```python
from build123d import *

# Parameters (mm, degrees)
BOSS_EXTRUDE1_DEPTH         = 12.7
SKETCH2_W                   = 323.85
SKETCH2_H                   = 152.4
CUT_EXTRUDE1_DEPTH          = 12.7
F_1_4_0_25_DIAMETER_HOLE1_D = 6.35
CUT_EXTRUDE2_DEPTH          = 13.7
SKETCH9_R                   = 3.175
CUT_EXTRUDE3_DEPTH          = 13.7
SKETCH10_R                  = 3.175
CUT_EXTRUDE4_DEPTH          = 13.7
LPATTERN1_COUNT             = 5
LPATTERN1_PITCH             = 25.4


with BuildPart() as part:
    # Sketch1 → Boss-Extrude1 (new body)
    with BuildSketch(Plane(origin=(0, 0, 0), x_dir=(0, 0, -1), z_dir=(1, 0, 0))):
        with BuildLine():
            Line((0, 609.6), (323.85, 609.6))
            Line((323.85, 609.6), (323.85, 0))
            Line((323.85, 0), (0, 0))
            Line((0, 0), (0, 31.75))
            ThreePointArc((0, 31.75), (188.340145046, 304.8), (0, 577.85))
            Line((0, 577.85), (0, 609.6))
        make_face()
    extrude(amount=BOSS_EXTRUDE1_DEPTH)

    # Sketch2 → Cut-Extrude1 (cut)
    with BuildSketch(Plane(origin=(12.7, 0, 0), x_dir=(0, 0, -1), z_dir=(1, 0, 0))):
        with Locations((161.925, 533.4)):
            Rectangle(SKETCH2_W, SKETCH2_H)
    extrude(amount=-CUT_EXTRUDE1_DEPTH, mode=Mode.SUBTRACT)

    # 1/4 (0.25) Diameter Hole1 (through all)
    with Locations(Plane(origin=(12.7, 0, 0), x_dir=(0, 0, -1), z_dir=(1, 0, 0))):
        with Locations((20.67422398, 12.7), (44.370645325, 23.973354386), (67.055185152, 37.165039515), (88.57288505, 52.184942803), (108.776757311, 68.93046308), (127.528789002, 87.287211463), (144.70088473, 107.129792746), (160.17574167, 128.32266198), (173.847650859, 150.721050378), (185.623219292, 174.171954236), (195.422007898, 198.515180102), (203.177081014, 223.584439059), (208.835463627, 249.208482649), (212.358503247, 275.212272671), (213.722133941, 301.418176873), (212.917040728, 327.647182356), (209.948723211, 353.720118416), (204.837458009, 379.458880463), (197.618160246, 404.687646654), (188.340145046, 429.234078933)):
            Hole(F_1_4_0_25_DIAMETER_HOLE1_D / 2)

    # Sketch8 → Cut-Extrude2 (cut, through all)
    with BuildSketch(Plane(origin=(12.7, 0, 0), x_dir=(0, 0, -1), z_dir=(1, 0, 0))):
        with BuildLine():
            Line((270.760801555, 457.2), (323.85, 457.2))
            Line((323.85, 457.2), (323.85, 0))
            Line((323.85, 0), (161.925, 0))
            ThreePointArc((161.925, 0), (289.589524386, 211.163746738), (270.760801555, 457.2))
        make_face()
    extrude(amount=-CUT_EXTRUDE2_DEPTH, mode=Mode.SUBTRACT)

    # Sketch9 → Cut-Extrude3 (cut, through all)
    with BuildSketch(Plane(origin=(12.7, 0, 0), x_dir=(0, 0, -1), z_dir=(1, 0, 0))):
        with Locations((214.065703753, 83.37972827)):
            Circle(SKETCH9_R)
        with Locations((277.383754924, 373.862081852)):
            Circle(SKETCH9_R)
    extrude(amount=-CUT_EXTRUDE3_DEPTH, mode=Mode.SUBTRACT)

    # Sketch10 → Cut-Extrude4 (cut, through all)
    with BuildSketch(Plane.ZY):
        with Locations((-154.03800305, 12.7)):
            Circle(SKETCH10_R)
    cut_extrude4 = extrude(amount=-CUT_EXTRUDE4_DEPTH, mode=Mode.SUBTRACT)

    # LPattern1: Cut-Extrude4 ×5
    with Locations(*[(0, 0, i * LPATTERN1_PITCH) for i in range(1, LPATTERN1_COUNT)]):
        add(cut_extrude4, mode=Mode.SUBTRACT)


solid = part.part
```
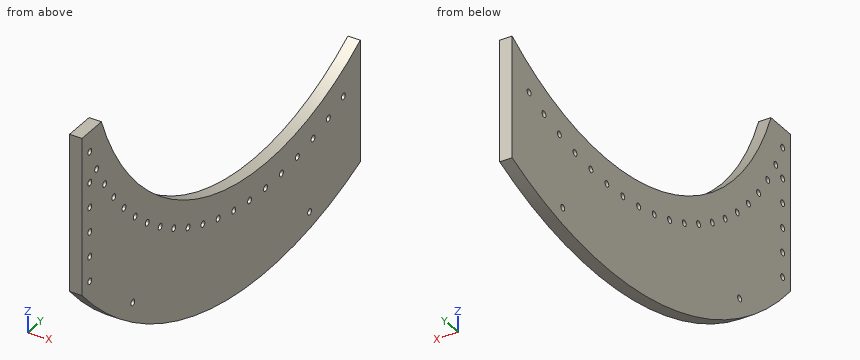
The model under review builds one solid part; all positions refer to its coordinate system, in mm. Round coordinates to 2 decimals unless told otherwise and drop trailing zeros. Write each loop counter-clockwise with the first axis right and the second up, starting at its lowest first coordinate (ties: lowest second). Pieces come first, ordered by that corner, then holes. Notation, with made-up numbers: (11, 5) - (33, 5) arc R23 cw to (33, 28) - close; hole circle Ø7 at (81, 89). An arc over 180 degrees is marked (long way). Answer as CSV lines item,"result". Start each with the question number.
(1) We need section A-A on x = 4.75. Give the number of separate pieces and of enclosed holes in the cut face, plus the area to 3 significant figures.
(2) We need section B-B on y = 293.5. State the section outline as (x, z) points, plus the area to 3 significant figures.
(3) For pin 1 Ø8.5 at (y, z) = (12.7, -128.64) entering from -X; pin 2 Ø1 at (x, z) = (3.5, -261) entering from -Y; pin 3 Ø1.5 at (x, y) = (8, 410) entering from +Z; pin 4 Ø1 at (x, z) = (3.5, -211.5) entering from -Y, all flat-tipped, find the tip position at first contact; note any pin that passes through.
(4) We need section C-C on y = 165. State the section outline as (x, z) points.
(5) To check wall thickness, follow line 1 (Y direction, x = 10, z = -20.5); line 2 (Y direction, x = 9.25, z = -91); line 3 (Z direction, x = 6, y = 308). State the ranges of each line that lie inside material, in increasing order.
Worked answers:
1,separate pieces,"1"
1,enclosed holes,"27"
1,area,"58,200 mm²"
2,outline,"(0, -300.42) - (12.7, -300.42) - (12.7, -188.12) - (0, -188.12) - close"
2,area,"1,430 mm²"
3,pin 1,"x = 0"
3,pin 2,"y = 129.28"
3,pin 3,"z = -168.45"
3,pin 4,"y = 50.99"
4,outline,"(0, -275.64) - (12.7, -275.64) - (12.7, -152.71) - (0, -152.71) - close"
5,line 1,"0 to 9.53, 15.87 to 40.45"
5,line 2,"0 to 50.14, 54.23 to 87.11"
5,line 3,"-300.57 to -188.32"
